Could you check a few things on this model? Use its own coordinates, in mm. A direction names the side the tool comes from. Coordinates: 2 decimals unless noted, no trailing zeros. Order: outer loops, then holes, each group sorted by start corner. A loop starts at its lowest first (then second) coordinate and runs counter-clockwise, first axis right, second up.
```python
from build123d import *

# Parameters (mm, degrees)
ESBO_O1_R          = 13
ESBO_O1_R_2        = 3.4
FLANGE_BASE1_DEPTH = 9.53


# Sheet-metal steps are written as plain solids
with BuildPart() as part:
    # Esboço1 → Flange-base1 (new body)
    with BuildSketch(Plane(origin=(0, 0, 0), x_dir=(1, 0, 0), z_dir=(0, 1, 0))):
        with BuildLine():
            Line((-59.5, -5), (59.5, -5))
            ThreePointArc((59.5, -5), (99.305049758, 1.425599896), (135.066417315, 20.049641099))
            ThreePointArc((135.066417315, 20.049641099), (170.049641099, 14.933582685), (164.933582685, -20.049641099))
            ThreePointArc((164.933582685, -20.049641099), (115.037752802, -46.034720952), (59.5, -55))
            Line((59.5, -55), (-59.5, -55))
            ThreePointArc((-59.5, -55), (-115.037752802, -46.034720952), (-164.933582685, -20.049641099))
            ThreePointArc((-164.933582685, -20.049641099), (-170.049641099, 14.933582685), (-135.066417315, 20.049641099))
            ThreePointArc((-135.066417315, 20.049641099), (-99.305049758, 1.425599896), (-59.5, -5))
        make_face()
        with Locations(Location((-150, 0, 0), (0, 0, 270))):
            Circle(ESBO_O1_R, mode=Mode.SUBTRACT)
        with Locations(Location((150, 0, 0), (0, 0, 270))):
            Circle(ESBO_O1_R, mode=Mode.SUBTRACT)
        with Locations(Location((-125.94, -17.92, 0), (0, 0, 270))):
            Circle(ESBO_O1_R_2, mode=Mode.SUBTRACT)
        with Locations(Location((125.94, -17.92, 0), (0, 0, 270))):
            Circle(ESBO_O1_R_2, mode=Mode.SUBTRACT)
    extrude(amount=-FLANGE_BASE1_DEPTH)


solid = part.part
```
Item 1: I need wall thicknesses on line 1 (X direction, y = -5.25, z = -9.5); line 2 (X direction, y = -6.75, z = 17.92); line 3 (X direction, y = -1.5, z = 7). Which ranges of each line are inside material? Lowest first, please.
Item 2: Suppose I cut it at C-C (x = 125.94). List the corners of the cut face in (y, z) for me, and give its area (3 significant figures).
Item 3: Suppose I cut it at D-D (z = 0). List the corners of the cut face in (x, y) for me.
Item 4: Suppose I cut it at A-A (z = -17). List the corners of the cut face in (x, y) for me.
Item 5: Suppose I cut it at B-B (y = -2). List the corners of the cut face in (x, z) for me, and give its area (3 significant figures).
Item 6: Thinking about a two-plate mould opening in X: for faces 3 (the face through (115.788, -4.698, 45.784)), 4 (the face through (2, 0, 23)), 5 (the face through (-114.29, -4.7, 46.28)), 6 (the face through (122.924, -4.698, 19.489)), which applies, +X half, -X half, draft (parallel to the pull), parting line (faces both ways), or undercut?
Item 7: For pin 1 Ø1 at (y, z) = (-2, 6) entering from -X; pin 2 Ø5 at (x, y) = (-107.5, -6) entering from +Z; pin 3 Ø5 at (x, y) = (-106, -5.5) entering from +Z, each with a flat end and sliding along its axis, tell me the tip position at first contact or that it passes through.
Item 8: Which directions (+Z, -Z, +X, -X, +Y, -Y) give clear straight access to the entire face, cutting with the end or side of a thin tool? Please do faces 1 (the face through (170, -5, -15)), 2 (the face through (98.77, -4.7, -1.25)).
Geometry results:
1. line 1: x = -173.12 to -158.87, -141.13 to -118.31, 118.31 to 141.13, 158.87 to 173.12
1. line 2: x = -167.43 to -129.34, -122.54 to 122.54, 129.34 to 167.43
1. line 3: x = -174 to -160.95, -139.05 to 139.05, 160.95 to 174
2. outline: (-9.53, -13.85) - (0, -13.85) - (0, 14.52) - (-9.53, 14.52) - close; (-9.53, 21.32) - (0, 21.32) - (0, 42.02) - (-9.53, 42.02) - close
2. area: 468 mm2
3. outline: (-175, -9.53) - (-163, -9.53) - (-163, 0) - (-175, 0) - close; (-137, -9.53) - (-94.71, -9.53) - (-94.71, 0) - (-137, 0) - close; (94.71, -9.53) - (137, -9.53) - (137, 0) - (94.71, 0) - close; (163, -9.53) - (175, -9.53) - (175, 0) - (163, 0) - close
4. outline: (-168.33, -9.53) - (-130.79, -9.53) - (-130.79, 0) - (-168.33, 0) - close; (130.79, -9.53) - (168.33, -9.53) - (168.33, 0) - (130.79, 0) - close
5. outline: (-164.93, 20.05) arc R25 ccw to (-135.07, -20.05) arc R126.5 cw to (-59.5, 5) - (59.5, 5) arc R126.5 cw to (135.07, -20.05) arc R25 ccw to (164.93, 20.05) arc R176.5 ccw to (59.5, 55) - (-59.5, 55) arc R176.5 ccw to start; hole circle Ø26 at (-150, 0); hole circle Ø6.8 at (-125.94, 17.92); hole circle Ø6.8 at (125.94, 17.92); hole circle Ø26 at (150, 0)
5. area: 16,500 mm2
6. face 3: +X half
6. face 4: draft
6. face 5: -X half
6. face 6: undercut
7. pin 1: stops at x = -174.39
7. pin 2: stops at z = 49.03
7. pin 3: stops at z = 49.43
8. face 1: +Y, -Y
8. face 2: -Z, +Y, -Y
